Geometry: final body of the model. Coordinates: model frame, mm. Face numbers are marked on the shaded views. A direction names the side the tool comes from. Give positions to 0.01 mm unless a question says otherwise; leave off trailing zeros. Order: outer loops, then holes, each group sorted by start corner. A loop starts at its lowest first (then second) coordinate and runs counter-clockwise, first axis right, second up. Notation, with made-up numbers: (-11.75, 84) - (47.25, 84) arc R26 ccw to (47.25, 116) - close; hole circle Ø6 at (52, 82.5). An arc over 180 degrees is marked (long way). Put each result on its own line as item: value. Start each with the question number.
1. Ray query, line 1 along X through (y, z) = (41, -3); line 2 along Y through (x, z) = (-9.25, 6); line 3 along Y through (x, z) = (-0.75, -5.25). Return the intervals inside material, ascending. Write a range as from..to.
2. Section C-C on z = -5.5. Return the cut outline in (x, y).
3. First-contact query: P1, Ø3, axis at x = -4.5, z = 4, coming from the +Y side; P2, Ø3, axis at x = -4, z = -4.5, coming from the -Y side; P3, Ø6, axis at y = -7, z = -1.5, coming from the -X side. Flat tips, straight axial feed; report the tip coordinate or a pass-through.
4. Set-up query: the marked faces 1, 2 and 3. Return all of +Z, -Z, +X, -X, +Y, -Y with unobstructed straight access to the full face (end or side cutting, diameter ignored); none if empty.
5. Section D-D on x = -6. Return the cut outline in (y, z).
6. Section A-A on z = 5.5. Return the cut outline in (x, y).
7. Section B-B on z = -0.5. Return the cut outline in (x, y).
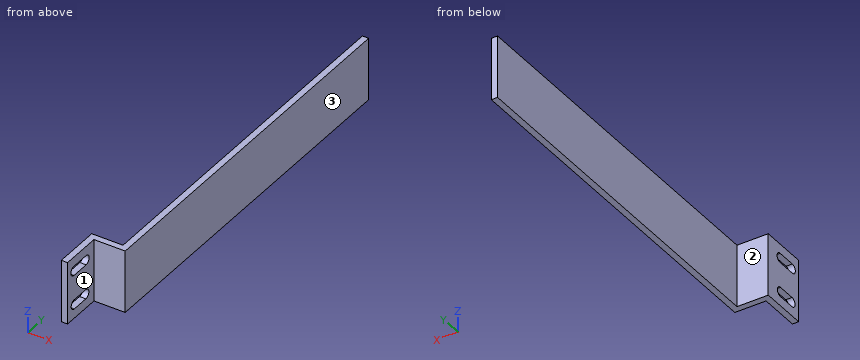
from build123d import *

# Parameters (mm, degrees)
F0_W     = 120
F0_H     = 20
F1_DEPTH = 2
F2_W     = 8
F2_H     = 20
F3_DEPTH = 2
F4_W     = 15
F4_H     = 20
F5_DEPTH = 2


with BuildPart() as f1:
    # F0 (on Right) → F1 (new body)
    with BuildSketch(Plane.YZ):
        Rectangle(F0_W, F0_H)
    extrude(amount=F1_DEPTH)

    # F2 (on face) → F3 (join)
    with BuildSketch(Plane.XZ.offset(60)):
        with Locations((-4, 0)):
            Rectangle(F2_W, F2_H)
    extrude(amount=-F3_DEPTH)

    # F4 (on face) → F5 (join)
    with BuildSketch(Plane(origin=(-8, 0, 0), x_dir=(0, -1, 0), z_dir=(-1, 0, 0))):
        with Locations((65.5, 0)):
            Rectangle(F4_W, F4_H)
        with BuildLine():
            Line((69.711817, -7), (63.999042, -7))
            ThreePointArc((63.999042, -7), (62.499042, -5.5), (63.999042, -4))
            Line((63.999042, -4), (69.711817, -4))
            ThreePointArc((69.711817, -4), (71.211817, -5.5), (69.711817, -7))
        make_face(mode=Mode.SUBTRACT)
        with BuildLine():
            Line((69.855429, 4), (63.855429, 4))
            ThreePointArc((63.855429, 4), (62.355429, 5.5), (63.855429, 7))
            Line((63.855429, 7), (69.855429, 7))
            ThreePointArc((69.855429, 7), (71.355429, 5.5), (69.855429, 4))
        make_face(mode=Mode.SUBTRACT)
    extrude(amount=F5_DEPTH)


solid = f1.part
Resolved:
1. line 1: 0..2
1. line 2: -73..-71.27, -62.44..-58
1. line 3: -60..-58
2. outline: (-10, -73) - (-8, -73) - (-8, -71.21) - (-10, -71.21) - close; (-10, -62.5) - (-8, -62.5) - (-8, -60) - (2, -60) - (2, 60) - (0, 60) - (0, -58) - (-10, -58) - close
3. P1: y = -58
3. P2: y = -60
3. P3: x = 0
4. face 1: +Z, -Z, +X, -Y
4. face 2: +Z, -Z, -X, +Y
4. face 3: +Z, -Z, +X, +Y, -Y
5. outline: (-60, -10) - (-58, -10) - (-58, 10) - (-60, 10) - close
6. outline: (-10, -73) - (-8, -73) - (-8, -71.36) - (-10, -71.36) - close; (-10, -62.36) - (-8, -62.36) - (-8, -60) - (2, -60) - (2, 60) - (0, 60) - (0, -58) - (-10, -58) - close
7. outline: (-10, -73) - (-8, -73) - (-8, -60) - (2, -60) - (2, 60) - (0, 60) - (0, -58) - (-10, -58) - close
